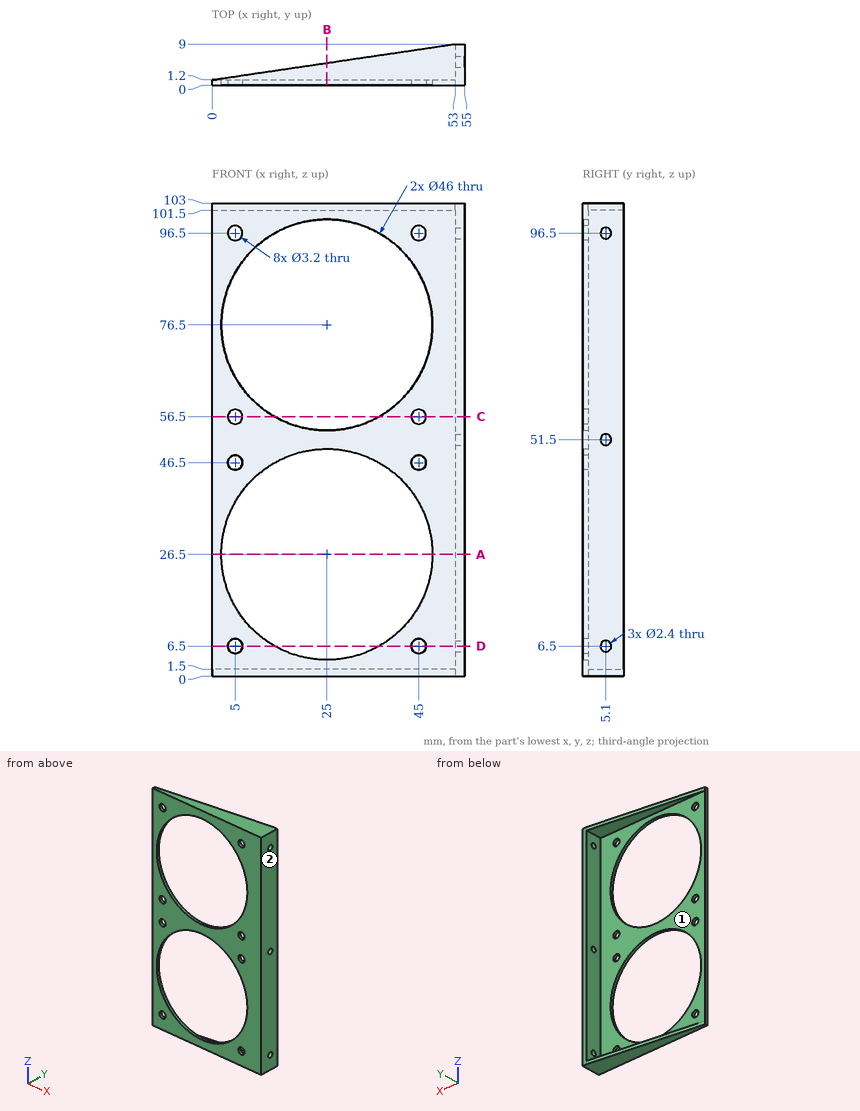
Geometry check sheet. Reference: drawing and pictorial views, mm from the part's lowest x, y, z. Round coordinates to 2 decimals unless told otherwise and drop trailing zeros. Order: outer loops, then holes, each group sorted by start corner. A loop starts at its lowest first (then second) coordinate and runs counter-clockwise, first axis right, second up.
Q1. Draft check along Z on the marked faces 1 and 2. Enter one of: pulls with the +Z half, pulls with the -Z half, needs draft (parallel to the pull), parting line crosses it, or undercut.
Filled sheet:
face 1: undercut
face 2: needs draft
Q2. Cross-section at B-B, the plane x = 25. Enter the section's corners in (y, z).
Filled sheet:
outline: (0, 0) - (4.88, 0) - (4.88, 1.5) - (1.2, 1.5) - (1.2, 3.5) - (0, 3.5) - close; (0, 49.5) - (1.2, 49.5) - (1.2, 53.5) - (0, 53.5) - close; (0, 99.5) - (1.2, 99.5) - (1.2, 101.5) - (4.88, 101.5) - (4.88, 103) - (0, 103) - close
Q3. Scan lines: L1, parallel to Z at x = 53.8, y = 5.1; L2, parallel to Z at x = 21.5, y = 1.5; L3, parallel to X at y = 0.75, z = 6.5. Record each from-to range of solid material in increasing order.
Filled sheet:
L1: z = 0 to 5.3, 7.7 to 50.3, 52.7 to 95.3, 97.7 to 103
L2: z = 0 to 1.5, 101.5 to 103
L3: x = 0 to 3.4, 6.6 to 13.64, 36.36 to 43.4, 46.6 to 55
Q4. Depth check by flat-ended pin: P1, Ø5, axis at x = 5, z = 56.5, coming from the +Y side; P2, Ø1.9, axis at x = 45, z = 6.5, coming from the +Y side; P3, Ø2, axis at y = 7.5, z = 57, coming from the -X side. Enter the tip coordinate at first touch or a pass-through.
Filled sheet:
P1: stops at y = 1.2
P2: passes through
P3: stops at x = 53
Q5. Cross-section at C-C, the plane z = 56.5. Enter the section's corners in (x, y), plus the area to 3 significant figures.
Filled sheet:
outline: (0, 0) - (3.4, 0) - (3.4, 1.2) - (0, 1.2) - close; (6.6, 0) - (13.64, 0) - (13.64, 1.2) - (6.6, 1.2) - close; (36.36, 0) - (43.4, 0) - (43.4, 1.2) - (36.36, 1.2) - close; (46.6, 0) - (55, 0) - (55, 9) - (53, 9) - (53, 1.2) - (46.6, 1.2) - close
area: 46.7 mm2
Q6. Cross-section at A-A, the plane z = 26.5. Enter the section's corners in (x, y), plus the area to 3 significant figures.
Filled sheet:
outline: (0, 0) - (2, 0) - (2, 1.2) - (0, 1.2) - close; (48, 0) - (55, 0) - (55, 9) - (53, 9) - (53, 1.2) - (48, 1.2) - close
area: 26.4 mm2
Q7. Cross-section at D-D, the plane z = 6.5. Enter the section's corners in (x, y), plus the area to 3 significant figures.
Filled sheet:
outline: (0, 0) - (3.4, 0) - (3.4, 1.2) - (0, 1.2) - close; (6.6, 0) - (13.64, 0) - (13.64, 1.2) - (6.6, 1.2) - close; (36.36, 0) - (43.4, 0) - (43.4, 1.2) - (36.36, 1.2) - close; (46.6, 0) - (55, 0) - (55, 3.9) - (53, 3.9) - (53, 1.2) - (46.6, 1.2) - close; (53, 6.3) - (55, 6.3) - (55, 9) - (53, 9) - close
area: 41.9 mm2
